Autodesk Inventor part; units mm, degrees
ref_plane "YZ Plane" through (0, 0, 0) normal (1, 0, 0) x (0, 1, 0)
ref_plane "XZ Plane" through (0, 0, 0) normal (0, 1, 0) x (-1, 0, 0)
ref_plane "XY Plane" through (0, 0, 0) normal (0, 0, 1) x (1, 0, 0)
sketch "Sketch1" plane through (0, 0, 0) normal (1, 0, 0) x (0, 1, 0)
  line L0 (3.4615, 28.4615) -> (-1.5385, 28.4615)
  line L1 (-1.5385, 28.4615) -> (-1.5385, -11.5385)
  line L2 (-1.5385, -11.5385) -> (3.4615, -11.5385)
  line L3 (3.4615, -11.5385) -> (3.4615, 28.4615)
  line L4 (3.4615, -11.5385) -> (-2.6923, -26.4744)
  line L5 (-2.8588, -26.8784) -> (-2.8558, -26.8796)
  line L6 (-2.8558, -26.8796) -> (-2.6923, -26.4744)
  line L7 (-2.8558, -26.8796) -> (-7.4503, -24.7123)
  line L8 (-7.4503, -24.7123) -> (-1.5385, -11.5385)
  point P0 (0, 0)
  dimension "d0" = 5
  dimension "d1" = 5.08
  dimension "d21" = 40
extrude "Extrusion1" add sketch "Sketch1" along normal blind 5
sketch "Sketch2" plane through (5, -2.8558, -26.8796) normal (0, -0.426635, -0.9044239) x (-1, 0, 0)
  circle A0 centre (2.5, -2.5) radius 2.0828
  line L0 (5, -5.08) -> (5, 0)
  line L1 (5, 0) -> (0, 0)
  point P0 (5, -8.885)
  dimension "d4" = 4.1656
  dimension "d5" = 2.5
  dimension "d6" = 2.5
extrude "Extrusion2" add sketch "Sketch2" along normal blind 30
sketch "Sketch7" plane through (2.5, -17.9159, -52.9458) normal (0, -0.426635, -0.9044239) x (-1, 0, 0)
  line L0 (2.5, -2.58) -> (-2.5, -2.58)
  line L1 (-2.5, 2.2849) -> (2.5, 2.2849)
  line L2 (2.5, 2.2849) -> (2.5, -2.58)
  line L3 (2.5, -2.58) -> (-2.5, -2.58)
  line L4 (-2.5, -2.58) -> (-2.5, 2.2849)
  point P0 (2.5, -6.385)
extrude "Extrusion3" add sketch "Sketch7" along normal blind 5
sketch "Sketch8" plane through (0, -20.2493, -51.8451) normal (-1, 0, 0) x (0, 0.426635, 0.9044239)
  circle A0 centre (-2.5, 2.3649) radius 2.0828
  line L0 (-5, 0) -> (-5, 4.8649)
  line L1 (0, 4.8649) -> (-5, 4.8649)
  point P0 (55.529, -3.805)
  dimension "d13" = 4.1656
  dimension "d14" = 2.5
  dimension "d15" = 2.5
extrude "Extrusion4" cut sketch "Sketch8" against normal blind 15
thread "Thread1"
fillet "Fillet1" radius 1 4 edges at (2.5, -22.3825, -56.3672) (2.5, -17.9826, -58.4427) (2.5, -15.8494, -53.9206) (2.5, -20.2493, -51.8451)
sketch "Sketch9" plane through (0, -20.6759, -52.7495) normal (0, -0.9044239, 0.426635) x (1, 0, 0)
  line L0 (0, -3.5828) -> (0, 0.5828)
  line L1 (5, 0) -> (5, -3)
  line L2 (0, 0.004) -> (5, 0.004)
  line L3 (5, 0.004) -> (5, -3)
  line L4 (5, -3) -> (0, -3)
  line L5 (0, -3) -> (0, 0.004)
  point P0 (0, 56.529)
extrude "Extrusion5" add sketch "Sketch9" along normal blind 1
sketch "Sketch10" plane through (0, -16.276, -54.825) normal (0, 0.9044239, -0.426635) x (1, 0, 0)
  point P0 (0, -56.529)
sketch "Sketch11" plane through (0, -16.276, -54.825) normal (0, 0.9044239, -0.426635) x (1, 0, 0)
  line L0 (5, -0.004) -> (5, -1)
  line L1 (0, 0) -> (0, 3)
  line L2 (5, -0.004) -> (0, -0.004)
  line L3 (0, -0.004) -> (0, 3)
  line L4 (0, 3) -> (5, 3)
  line L5 (5, 3) -> (5, -0.004)
  point P0 (0, -56.529)
extrude "Extrusion6" add sketch "Sketch11" along normal blind 1
properties part number "Fingers IPT"
Geometry: final body of the model. Coordinates: model frame, mm. A direction names the side the tool comes from. Give positions to 0.01 mm unless a question says otherwise; leave off trailing zeros. Write each loop counter-clockwise with the first axis right and the second up, starting at its lowest first coordinate (ties: lowest second). Pieces come first, ordered by that corner, then holes. Notation, with made-up numbers: (71.5, 8.5) -> (109.5, 8.5) arc R17 cw to (109.5, 14.5) -> close; hole circle Ø7 at (86.5, -24). An arc over 180 degrees is marked (long way). Answer in a Markdown table with one row per item.
(1) Draft query along Y for faces 1 (the flat face through (2, 3.462, 8)), 2 (the flat face through (0.24, -5.12, -25.81)), 3 (the flat face through (5, -20.1, -57.2)). Return one class per face: +Y half, -Y half, draft (parallel to the pull), parting line (faces both ways), or undercut.
Answers below:
| item | result |
|---|---|
| face 1 | +Y half |
| face 2 | undercut |
| face 3 | draft |
(2) Section query C-C on y = -0.75. Return loops of the section in (x, z), then the cut area to 3 significant figures.
Answers below:
| item | result |
|---|---|
| outline | (0, -21.76) -> (5, -21.76) -> (5, 28.46) -> (0, 28.46) -> close |
| area | 251 mm^2 |
(3) Section query B-B on z = 23. Return loops of the section in (x, y), then the cut area to 3 significant figures.
Answers below:
| item | result |
|---|---|
| outline | (0, -1.54) -> (5, -1.54) -> (5, 3.46) -> (0, 3.46) -> close |
| area | 25.0 mm^2 |
(4) Pin query (flat end, axial travel): pin 1 (2.5 mm diameter, centred on y = -19.18, z = -55.12, fed in from -X); pin 2 (1.5 mm diameter, centred on x = 2, z = 5.5, fed in from -Y); pin 3 (2 mm diameter, centred on x = 4, z = -43, fed in from -Y); pin 4 (12 mm diameter, centred on y = -7, z = -7.5, fed in from -X). Return the tip coordinate at first contact, or that it passes through.
Answers below:
| item | result |
|---|---|
| pin 1 | through |
| pin 2 | y = -1.54 |
| pin 3 | y = -15.69 |
| pin 4 | x = 0 |
(5) Ray query, line 1 along Z through (x, y) = (1.65, 0.25); line 2 along Y through (x, z) = (1.9, 5.5); line 3 along Z through (x, y) = (2.9, -19). Return the intervals inside material, ascending. Write a range as [from, to].
Answers below:
| item | result |
|---|---|
| line 1 | [-19.33, 28.46] |
| line 2 | [-1.54, 3.46] |
| line 3 | [-57.96, -57.19], [-53.04, -50.45] |
(6) Set-up query: faces 4 (the flat face through (2, -1.538, 9)), 5 (the flat face through (2.47, -16.02, -56.63)). Return all of +Z, -Z, +X, -X, +Y, -Y with unobstructed straight access to the full face (end or side cutting, diameter ignored); none if empty.
Answers below:
| item | result |
|---|---|
| face 4 | +Z, +X, -X, -Y |
| face 5 | -Z, +X, -X, +Y |
